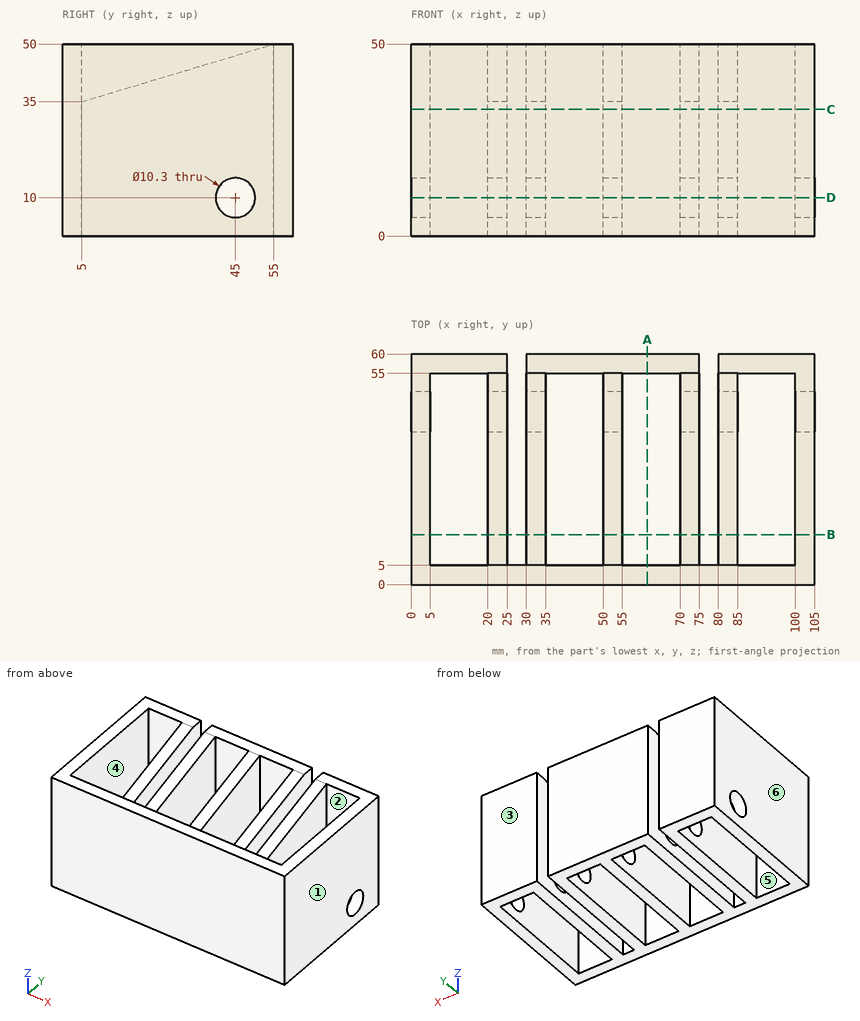
Drawing for the job (mm, zero at the part's lowest x, y, z). A direction names the side the tool comes from. Give positions to 0.01 mm unless a question says otherwise; leave off trailing zeros. Order: outer loops, then holes, each group sorted by start corner. A loop starts at its lowest first (then second) coordinate and runs counter-clockwise, first axis right, second up. Notation, with made-up numbers: M -14,70 L 36,70 A32 cw 36,101 Z; hole C 35,11 d3. An arc over 180 degrees is marked long. Put each result on its own line as item: value.
Item 1: 3-axis set-ups, long thin cutter, end or side, ignore diameter. For the marked faces 4, 5 and 6: which of +Z, -Z, +X, -X, +Y, -Y reach the whole face in a straight line?
From the geometry:
face 4: +Z, -Z
face 5: +Z
face 6: +Z, -Z, -X, +Y, -Y
Item 2: Slice it at A-A, the plane x = 61.5. Write the cut outline in (y, z), plus the area to 3 significant figures.
From the geometry:
outline: M 0,0 L 5,0 L 5,50 L 0,50 Z; M 55,0 L 60,0 L 60,50 L 55,50 Z
area: 500 mm2
Item 3: Flat gauge pins, fed straight in: pin 1 Ø1.5 at (x, z) = (19, 24) entering from -Y; pin 2 Ø12 at (x, y) = (55, 32) entering from +Z. Where does each tip first touch, or does it go through?
From the geometry:
pin 1: stops at y = 0
pin 2: stops at z = 44.9
Item 4: Slice it at C-C, the plane z = 33. Write the cut outline in (x, y).
From the geometry:
outline: M 0,0 L 105,0 L 105,60 L 80,60 L 80,5 L 75,5 L 75,60 L 30,60 L 30,5 L 25,5 L 25,60 L 0,60 Z; hole M 5,5 L 20,5 L 20,55 L 5,55 Z; hole M 35,5 L 50,5 L 50,55 L 35,55 Z; hole M 55,5 L 70,5 L 70,55 L 55,55 Z; hole M 85,5 L 100,5 L 100,55 L 85,55 Z
Item 5: Probe line 1 (X direction, y = 56, z = 20.5); line 2 (Y direction, x = 46, z = 12.5); line 3 (X direction, y = 15.5, z = 45.5). List the from-to ranges inside material, lowest first. Write a range as [from, to].
From the geometry:
line 1: x = [0, 25], [30, 75], [80, 105]
line 2: y = [0, 5], [55, 60]
line 3: x = [0, 5], [100, 105]
Item 6: Two-plate mould, pull along Y, no slides. Class the marked faces 1, 2 and 3: +Y half, -Y half, draft (parallel to the pull), parting line (faces both ways), or undercut.
From the geometry:
face 1: draft
face 2: undercut
face 3: +Y half
Item 7: Slice it at B-B, the plane y = 13. Write the cut outline in (x, z), plus the area to 4 significant figures.
From the geometry:
outline: M 0,0 L 5,0 L 5,50 L 0,50 Z; M 20,0 L 25,0 L 25,37.4 L 20,37.4 Z; M 30,0 L 35,0 L 35,37.4 L 30,37.4 Z; M 50,0 L 55,0 L 55,37.4 L 50,37.4 Z; M 70,0 L 75,0 L 75,37.4 L 70,37.4 Z; M 80,0 L 85,0 L 85,37.4 L 80,37.4 Z; M 100,0 L 105,0 L 105,50 L 100,50 Z
area: 1,435 mm2
Item 8: Slice it at D-D, the plane z = 10. Give the number of separate pieces and of enclosed holes in the cut face, plus the area to 3 significant figures.
From the geometry:
separate pieces: 4
enclosed holes: 0
area: 2,390 mm2
